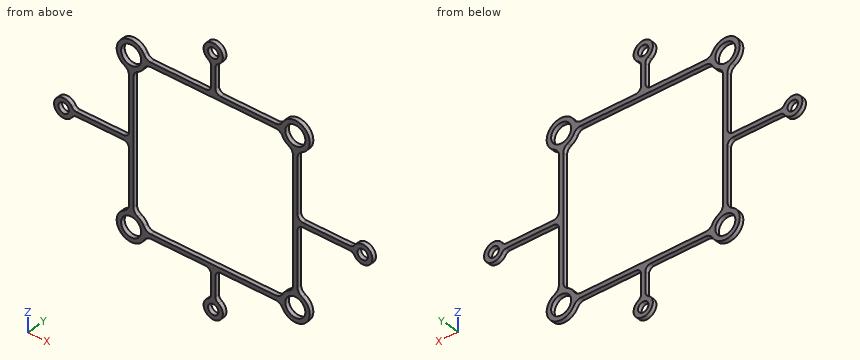
```python
from build123d import *

# Parameters (mm, degrees)
SKETCH1_R           = 3.71
SKETCH1_R_2         = 1.925
BOSS_EXTRUDE1_DEPTH = 1.5875
FILLET1_R           = 3
FILLET2_R           = 2
FILLET3_R           = 2


with BuildPart() as part:
    # Sketch1 → Boss-Extrude1 (new body)
    with BuildSketch(Plane(origin=(0, 0, 0), x_dir=(1, 0, 0), z_dir=(0, 1, 0))):
        with BuildLine():
            Line((-25.148871697, 31.27), (-0.825, 31.27))
            Line((-0.825, 31.27), (-0.825, 41.966494574))
            ThreePointArc((-0.825, 41.966494574), (0, 49.02), (0.825, 41.966494574))
            Line((0.825, 41.966494574), (0.825, 31.27))
            Line((0.825, 31.27), (25.148871697, 31.27))
            ThreePointArc((25.148871697, 31.27), (34.235092347, 34.235092347), (31.27, 25.148871697))
            Line((31.27, 25.148871697), (31.27, 0.825))
            Line((31.27, 0.825), (51.966494574, 0.825))
            ThreePointArc((51.966494574, 0.825), (59.02, 0), (51.966494574, -0.825))
            Line((51.966494574, -0.825), (31.27, -0.825))
            Line((31.27, -0.825), (31.27, -25.148871697))
            ThreePointArc((31.27, -25.148871697), (34.235092347, -34.235092347), (25.148871697, -31.27))
            Line((25.148871697, -31.27), (0.825, -31.27))
            Line((0.825, -31.27), (0.825, -41.966494574))
            ThreePointArc((0.825, -41.966494574), (0, -49.02), (-0.825, -41.966494574))
            Line((-0.825, -41.966494574), (-0.825, -31.27))
            Line((-0.825, -31.27), (-25.148871697, -31.27))
            ThreePointArc((-25.148871697, -31.27), (-34.235092347, -34.235092347), (-31.27, -25.148871697))
            Line((-31.27, -25.148871697), (-31.27, -0.825))
            Line((-31.27, -0.825), (-51.966494574, -0.825))
            ThreePointArc((-51.966494574, -0.825), (-59.02, 0), (-51.966494574, 0.825))
            Line((-51.966494574, 0.825), (-31.27, 0.825))
            Line((-31.27, 0.825), (-31.27, 25.148871697))
            ThreePointArc((-31.27, 25.148871697), (-34.235092347, 34.235092347), (-25.148871697, 31.27))
        make_face()
        with Locations(Location((-30.445, 30.445, 0), (0, 0, 270))):
            Circle(SKETCH1_R, mode=Mode.SUBTRACT)
        with Locations(Location((30.445, 30.445, 0), (0, 0, 90))):
            Circle(SKETCH1_R, mode=Mode.SUBTRACT)
        with Locations(Location((30.445, -30.445, 0), (0, 0, 270))):
            Circle(SKETCH1_R, mode=Mode.SUBTRACT)
        with Locations(Location((-30.445, -30.445, 0), (0, 0, 90))):
            Circle(SKETCH1_R, mode=Mode.SUBTRACT)
        with Locations(Location((0, 45.445, 0), (0, 0, 270))):
            Circle(SKETCH1_R_2, mode=Mode.SUBTRACT)
        with Locations(Location((55.445, 0, 0), (0, 0, 270))):
            Circle(SKETCH1_R_2, mode=Mode.SUBTRACT)
        with Locations(Location((0, -45.445, 0), (0, 0, 90))):
            Circle(SKETCH1_R_2, mode=Mode.SUBTRACT)
        with Locations(Location((-55.445, 0, 0), (0, 0, 90))):
            Circle(SKETCH1_R_2, mode=Mode.SUBTRACT)
        with BuildLine():
            Line((-25.148871697, 29.62), (25.148871697, 29.62))
            ThreePointArc((25.148871697, 29.62), (26.654907653, 26.654907653), (29.62, 25.148871697))
            Line((29.62, 25.148871697), (29.62, -25.148871697))
            ThreePointArc((29.62, -25.148871697), (26.654907653, -26.654907653), (25.148871697, -29.62))
            Line((25.148871697, -29.62), (-25.148871697, -29.62))
            ThreePointArc((-25.148871697, -29.62), (-26.654907653, -26.654907653), (-29.62, -25.148871697))
            Line((-29.62, -25.148871697), (-29.62, 25.148871697))
            ThreePointArc((-29.62, 25.148871697), (-26.654907653, 26.654907653), (-25.148871697, 29.62))
        make_face(mode=Mode.SUBTRACT)
    extrude(amount=BOSS_EXTRUDE1_DEPTH)

    # Fillet1
    fillet1_edges = [part.edges().sort_by_distance(p)[0] for p in [
        (25.148871697, 0.79375, -31.27),
        (31.27, 0.79375, -25.148871697),
        (31.27, 0.79375, 25.148871697),
        (25.148871697, 0.79375, 31.27),
        (-25.148871697, 0.79375, 31.27),
        (-31.27, 0.79375, 25.148871697),
        (-31.27, 0.79375, -25.148871697),
        (-25.148871697, 0.79375, -31.27),
        (-25.148871697, 0.79375, -29.62),
        (-29.62, 0.79375, -25.148871697),
        (-29.62, 0.79375, 25.148871697),
        (-25.148871697, 0.79375, 29.62),
        (25.148871697, 0.79375, 29.62),
        (29.62, 0.79375, 25.148871697),
        (29.62, 0.79375, -25.148871697),
        (25.148871697, 0.79375, -29.62),
    ]]
    fillet(fillet1_edges, radius=FILLET1_R)

    # Fillet2
    fillet2_edges = [part.edges().sort_by_distance(p)[0] for p in [
        (0.825, 0.79375, -31.27),
        (31.27, 0.79375, -0.825),
        (31.27, 0.79375, 0.825),
        (0.825, 0.79375, 31.27),
        (-0.825, 0.79375, 31.27),
        (-31.27, 0.79375, 0.825),
        (-31.27, 0.79375, -0.825),
        (-0.825, 0.79375, -31.27),
    ]]
    fillet(fillet2_edges, radius=FILLET2_R)

    # Fillet3
    fillet3_edges = [part.edges().sort_by_distance(p)[0] for p in [
        (0.825, 0.79375, -41.966494574),
        (51.966494574, 0.79375, -0.825),
        (51.966494574, 0.79375, 0.825),
        (0.825, 0.79375, 41.966494574),
        (-0.825, 0.79375, 41.966494574),
        (-51.966494574, 0.79375, 0.825),
        (-51.966494574, 0.79375, -0.825),
        (-0.825, 0.79375, -41.966494574),
    ]]
    fillet(fillet3_edges, radius=FILLET3_R)


solid = part.part
```
For this review, take the finished solid that the model builds, in its own axes (mm). Give positions to 0.01 mm unless a question says otherwise; leave off trailing zeros. Write each loop counter-clockwise with the first axis right and the second up, starting at its lowest first coordinate (ties: lowest second). Pieces come first, ordered by that corner, then holes. Notation, with made-up numbers: M 64.5,80 L 75.5,80 A22 ccw 75.5,97 Z; hole C 26,61.5 d5. An arc over 180 degrees is marked long. Answer as CSV lines item,"result".
1. Consider section B-B, the plane x = -44. Write out the cut boundary in (y, z) (1 decimal).
Findings:
outline,"M 0,-0.8 L 1.6,-0.8 L 1.6,0.8 L 0,0.8 Z"
2. Consider section A-A, the plane x = 15. Write out the cut boundary in (y, z), then the cut area to 3 significant figures.
Findings:
outline,"M 0,-31.27 L 1.59,-31.27 L 1.59,-29.62 L 0,-29.62 Z; M 0,29.62 L 1.59,29.62 L 1.59,31.27 L 0,31.27 Z"
area,"5.24 mm2"
3. Wall thickness on line 1 (X direction, y = 0.4, z = 0); line 2 (Z direction, x = 22.5, y = 1.5): over which ranges is each line inside the solid? List them lowest first.
Findings:
line 1,"x = -59.02 to -57.37, -53.52 to -29.62, 29.62 to 53.52, 57.37 to 59.02"
line 2,"z = -31.27 to -29.62, 29.62 to 31.27"
4. For pin 1 (0.5 mm diameter, centred on y = 0.5, z = 9.5, fed in from +X); pin 2 (0.5 mm diameter, centred on y = 0.5, z = 37.5, fed in from +X) (3 decimals); pin 3 (5 mm diameter, centred on x = -55.445, z = 0, fed in from +Y); pin 4 (0.5 mm diameter, centred on x = 9.5, y = 1, fed in from -Z), all flat-tipped, find the tip position at first contact; note any pin that passes through.
Findings:
pin 1,"stops at x = 31.27"
pin 2,"stops at x = 0.825"
pin 3,"stops at y = 1.59"
pin 4,"stops at z = -31.27"
5. Consider section C-C, the plane y = 0.8. Count the separate pieces of the cut face and the enclosed holes in it, then the cut area to 3 significant figures.
Findings:
separate pieces,"1"
enclosed holes,"9"
area,"757 mm2"
